Source: three-view drawing plus pictorial views. Frame: mm from the lowest corner of the part. A direction names the side the tool comes from. Give positions to 0.01 mm unless a question says otherwise; leave off trailing zeros. Loops run counter-clockwise (first coordinate to the right, second up) from the corner with the lowest first, then second, coordinate; pieces in that order, holes last. Notation, with made-up numbers: (-17, 18.5) - (17, 18.5) arc R27 cw to (17, 48.5) - close; hole circle Ø10 at (12.5, 64). An arc over 180 degrees is marked (long way). Answer in a Markdown table with one row per item.
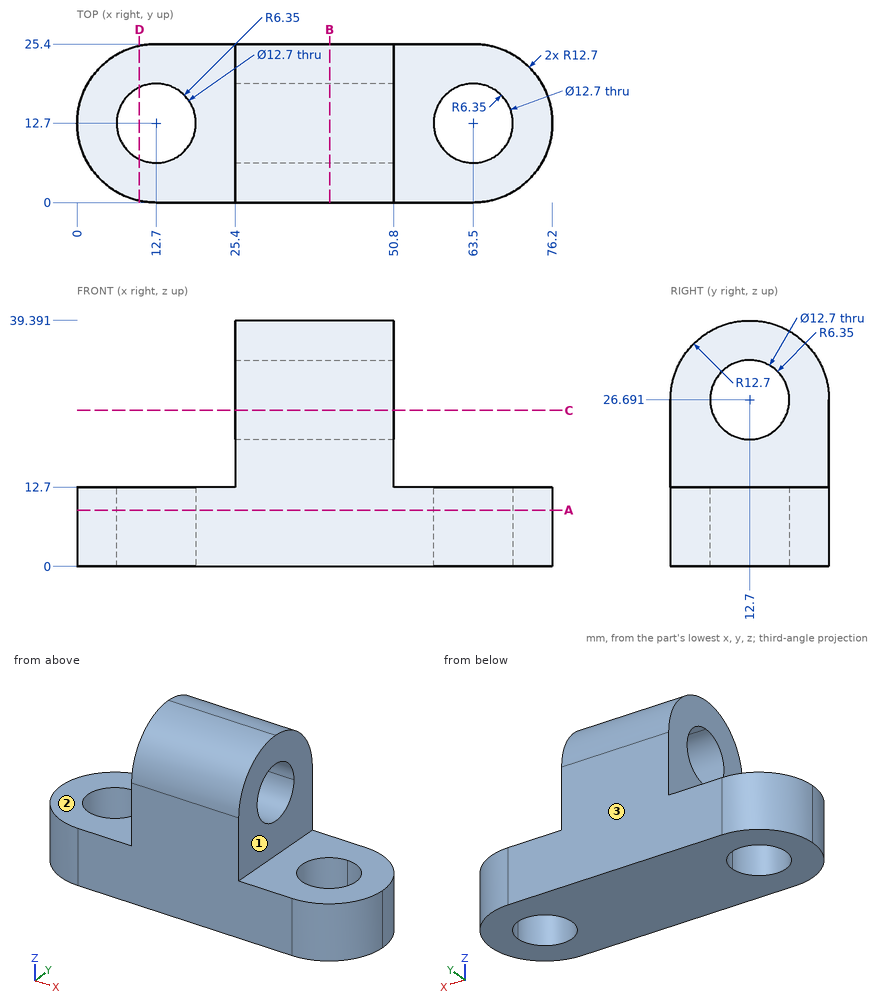
Q1. Cut plane A-A (z = 9). Output: boundary loops of the cut face in (x, y).
Check values:
| item | result |
|---|---|
| outline | (12.7, 0) - (63.5, 0) arc R12.7 ccw to (63.5, 25.4) - (12.7, 25.4) arc R12.7 ccw to start; hole circle Ø12.7 at (12.7, 12.7); hole circle Ø12.7 at (63.5, 12.7) |
Q2. First-contact query: pin 1 (3 mm diameter, centred on x = 14, y = 2.5, fed in from +Z); pin 2 (8 mm diameter, centred on y = 2.5, z = 27, fed in from +X); pin 3 (7.5 mm diameter, centred on y = 10, z = 28, fed in from -X). Flat tips, straight axial feed; report the tip coordinate or a pass-through.
Check values:
| item | result |
|---|---|
| pin 1 | z = 12.7 |
| pin 2 | x = 50.8 |
| pin 3 | x = 25.4 |
Q3. Material intervals for line 1 along Y through (x, z) = (12.7, 7); line 2 along X through (y, z) = (11.5, 8.5); line 3 along X through (y, z) = (18.5, 5.5) (1 decimal), sorted ascending.
Check values:
| item | result |
|---|---|
| line 1 | 0 to 6.35, 19.05 to 25.4 |
| line 2 | 0.06 to 6.46, 18.94 to 57.26, 69.74 to 76.14 |
| line 3 | 1.4 to 10.1, 15.3 to 60.9, 66.1 to 74.8 |
Q4. Cut plane B-B (x = 40.5). Output: boundary loops of the cut face in (y, z), and give its area (3 significant figures).
Check values:
| item | result |
|---|---|
| outline | (0, 0) - (25.4, 0) - (25.4, 26.69) arc R12.7 ccw to (12.7, 39.39) arc R12.7 ccw to (0, 26.69) - close; hole (12.59, 33.04) arc R6.35 ccw (long way) to (19.05, 26.69) arc R6.35 ccw to start |
| area | 805 mm² |
Q5. Reachability of the marked faces 1, 2 and 3 from +Z, -Z, +X, -X, +Y, -Y: full face, straight path, thin tool, end or side. Return the list, or none.
Check values:
| item | result |
|---|---|
| face 1 | +Z, +X, +Y, -Y |
| face 2 | +Z, -X, +Y, -Y |
| face 3 | +Z, -Z, +X, -X, +Y |
Q6. Cut plane D-D (x = 10). Output: boundary loops of the cut face in (y, z).
Check values:
| item | result |
|---|---|
| outline | (0.29, 0) - (6.95, 0) - (6.95, 12.7) - (0.29, 12.7) - close; (18.45, 0) - (25.11, 0) - (25.11, 12.7) - (18.45, 12.7) - close |
Q7. Cut plane C-C (z = 25). Output: boundary loops of the cut face in (x, y), and give its area (3 significant figures).
Check values:
| item | result |
|---|---|
| outline | (25.4, 0) - (50.8, 0) - (50.8, 6.58) - (25.4, 6.58) - close; (25.4, 18.82) - (50.8, 18.82) - (50.8, 25.4) - (25.4, 25.4) - close |
| area | 334 mm² |
